```python
from build123d import *

# Parameters (mm, degrees)
SKETCH1_W                = 20.5
SKETCH1_H                = 16.5
SKETCH1_W_2              = 14.5
SKETCH1_H_2              = 10.5
BOSS_EXTRUDE1_DEPTH      = 41.5
SKETCH2_W                = 14.5
SKETCH2_H                = 3
CUT_EXTRUDE1_DEPTH       = 15
BOSS_EXTRUDE2_DEPTH      = 50
BOSS_EXTRUDE2_DEPTH_BACK = 20
SKETCH5_R                = 2
CUT_EXTRUDE2_DEPTH       = 25
SKETCH12_W               = 7.15
SKETCH12_H               = 20
BOSS_EXTRUDE16_DEPTH     = 16.5
SKETCH13_W               = 3
SKETCH13_H               = 20
CUT_EXTRUDE5_DEPTH       = 12
CHAMFER1_SIZE            = 3
FILLET6_R                = 15
FILLET7_R                = 5
SKETCH7_R                = 2
CUT_EXTRUDE6_DEPTH       = 78.232603305
FILLET14_R               = 1


with BuildPart() as part:
    # Sketch1 → Boss-Extrude1 (new body)
    with BuildSketch(Plane.XY):
        Rectangle(SKETCH1_W, SKETCH1_H)
        Rectangle(SKETCH1_W_2, SKETCH1_H_2, mode=Mode.SUBTRACT)
    extrude(amount=BOSS_EXTRUDE1_DEPTH)

    # Sketch2 → Cut-Extrude1 (cut)
    with BuildSketch(Plane.XY.offset(41.5)):
        with Locations((0, 6.75)):
            Rectangle(SKETCH2_W, SKETCH2_H)
        with Locations((0, -6.75)):
            Rectangle(SKETCH2_W, SKETCH2_H)
    extrude(amount=-CUT_EXTRUDE1_DEPTH, mode=Mode.SUBTRACT)

    # Sketch3 → Boss-Extrude2 (add, two sides: drawn at the far end of the back side and taken through both)
    with BuildSketch(Plane(origin=(0, 0, 0), x_dir=(0, 0, -1), z_dir=(1, 0, 0)).offset(-BOSS_EXTRUDE2_DEPTH_BACK)):
        with BuildLine():
            Line((-13.882285677, -14.488887394), (-12.588190451, -9.659258263))
            ThreePointArc((-12.588190451, -9.659258263), (0, 0), (-12.588190451, 9.659258263))
            Line((-12.588190451, 9.659258263), (-13.882285677, 14.488887394))
            ThreePointArc((-13.882285677, 14.488887394), (5, 0), (-13.882285677, -14.488887394))
        make_face()
    extrude(amount=BOSS_EXTRUDE2_DEPTH + BOSS_EXTRUDE2_DEPTH_BACK)

    # Sketch5 → Cut-Extrude2 (cut)
    with BuildSketch(Plane(origin=(10.25, 0, 0), x_dir=(0, 0, -1), z_dir=(1, 0, 0))):
        with Locations(Location((-20, 0, 0), (0, 0, 90))):
            Circle(SKETCH5_R)
        with Locations(Location((-11, 0, 0), (0, 0, 90))):
            Circle(SKETCH5_R)
    extrude(amount=-CUT_EXTRUDE2_DEPTH, mode=Mode.SUBTRACT)

    # Sketch12 → Boss-Extrude16 (add)
    with BuildSketch(Plane.XZ.offset(8.25)):
        with Locations((-6.675, 31.5)):
            Rectangle(SKETCH12_W, SKETCH12_H)
        with Locations((6.675, 31.5)):
            Rectangle(SKETCH12_W, SKETCH12_H)
    extrude(amount=BOSS_EXTRUDE16_DEPTH)

    # Sketch13 → Cut-Extrude5 (cut)
    with BuildSketch(Plane.XZ.offset(24.75)):
        with Locations((-8.75, 31.5)):
            Rectangle(SKETCH13_W, SKETCH13_H)
        with Locations((8.75, 31.5)):
            Rectangle(SKETCH13_W, SKETCH13_H)
    extrude(amount=-CUT_EXTRUDE5_DEPTH, mode=Mode.SUBTRACT)

    # Chamfer1
    chamfer1_edges = [part.edges().sort_by_distance(p)[0] for p in [
        (7.25, -12.75, 31.5),
        (-7.25, -12.75, 31.5),
    ]]
    chamfer(chamfer1_edges, length=CHAMFER1_SIZE - 0.0001)  # a hair under: the kernel refuses the full size

    # Fillet6
    fillet6_edges = [part.edges().sort_by_distance(p)[0] for p in [
        (6.675, -8.25, 21.5),
        (-6.675, -8.25, 21.5),
    ]]
    fillet(fillet6_edges, radius=FILLET6_R)

    # Fillet7
    fillet7_edges = [part.edges().sort_by_distance(p)[0] for p in [
        (8.75, 8.25, 41.5),
        (-8.75, 8.25, 41.5),
        (5.175, -24.75, 21.5),
        (5.175, -24.75, 41.5),
        (-5.175, -24.75, 41.5),
        (-5.175, -24.75, 21.5),
    ]]
    fillet(fillet7_edges, radius=FILLET7_R)

    # Sketch7 → Cut-Extrude6 (cut, through all)
    with BuildSketch(Plane.ZY.offset(10.25)):
        with Locations(Location((34.590169944, -20, 0), (0, 0, 180))):
            Circle(SKETCH7_R)
    extrude(amount=-CUT_EXTRUDE6_DEPTH, mode=Mode.SUBTRACT)

    # Fillet14
    fillet14_edges = [part.edges().sort_by_distance(p)[0] for p in [
        (10.25, 0, 0),
        (-10.25, 0, 0),
    ]]
    fillet(fillet14_edges, radius=FILLET14_R)


solid = part.part
```
Work out the finished part from the listing and answer in its coordinate system (mm). A direction names the side the tool comes from. Round coordinates to 2 decimals unless told otherwise and drop trailing zeros. Order: outer loops, then holes, each group sorted by start corner. A loop starts at its lowest first (then second) coordinate and runs counter-clockwise, first axis right, second up.
Q1. Given pin 1 Ø7 at (y, z) = (-19, 26.5) entering from +X; pin 2 Ø1.5 at (x, y) = (33.5, -10) entering from +Z; pin 3 Ø4.5 at (y, z) = (0, 11) entering from +X; pin 4 Ø23 at (y, z) = (-3, 12) entering from -X, each flat-ended and moving along its own axis, determine where each tip first touches the part or whether it passes through.
Solution:
pin 1: stops at x = 7.5
pin 2: stops at z = 12.88
pin 3: stops at x = 10.25
pin 4: stops at x = -20
Q2. A cutting plane is placed at A-A, the plane z = 8. Determine the outline of the cut face in (x, y).
Solution:
outline: (-20, -14.87) - (50, -14.87) - (50, -9.8) - (-20, -9.8) - close; (-20, 9.8) - (50, 9.8) - (50, 14.87) - (-20, 14.87) - close; (-10.25, -8.33) - (-3.1, -8.33) - (-3.1, -8.25) - (3.1, -8.25) - (3.1, -8.33) - (10.25, -8.33) - (10.25, 8.25) - (-10.25, 8.25) - close; hole (-7.25, -5.25) - (7.25, -5.25) - (7.25, 5.25) - (-7.25, 5.25) - close
Q3. A cutting plane is placed at B-B, the plane y = 0. Count the separate pieces of the cut face and the enclosed holes in it, then the cut area to 3 significant figures.
Solution:
separate pieces: 5
enclosed holes: 0
area: 551 mm2
Q4. A cutting plane is placed at C-C, the plane x = -1.5. Determine the outline of the cut face in (y, z), then the cut area to 3 significant figures.
Solution:
outline: (-14.49, 13.88) arc R15 ccw (long way) to (14.49, 13.88) - (9.66, 12.59) arc R10 cw to (8.25, 4.35) - (8.25, 26.5) - (5.25, 26.5) - (5.25, 1.49) arc R10 cw to (-5.25, 1.49) - (-5.25, 26.5) - (-8.25, 26.5) - (-8.25, 4.35) arc R10 cw to (-9.66, 12.59) - close
area: 372 mm2
Q5. The mould has two halves that part along Y. Classify faces 5 (the cylindrical face through (6.73, -10.33, 14.12)), 6 (the flat face through (5, -24.75, 31)), 7 (the flat face through (5, -8.25, 34)): pulls with the +Y half, pulls with the -Y half, needs draft (parallel to the pull), parting line crosses it, or undercut.
Solution:
face 5: undercut
face 6: pulls with the -Y half
face 7: pulls with the +Y half
Q6. Find the intervals of material crossed by line 1 along X through (y, z) = (-7, 35); line 2 along Y through (x, z) = (2, 7.5); line 3 along Z through (x, y) = (-9, 0), in increasing order.
Solution:
line 1: x = -10.25 to -7.25, 7.25 to 10.25
line 2: y = -14.79 to -9.68, -8.25 to -5.25, 5.25 to 8.25, 9.68 to 14.79
line 3: z = -5 to 9, 13 to 18, 22 to 41.5
Q7. A tool of negligible diameter and unlimited length cuts with its end or side. For faces 1 (the flat face through (14.51, -12.108, 13.244)), 2 (the flat face through (0, -7, 26.5)), 3 (the flat face through (9, -14, 29)), 4 (the flat face through (0, 5.25, 14)), from which of +Z, -Z, +X, -X, +Y, -Y can it reach the whole face along a straight path? Write none if from no direction.
Solution:
face 1: +X, -X
face 2: +Z, +Y
face 3: +Z, +X, -Y
face 4: +Z
